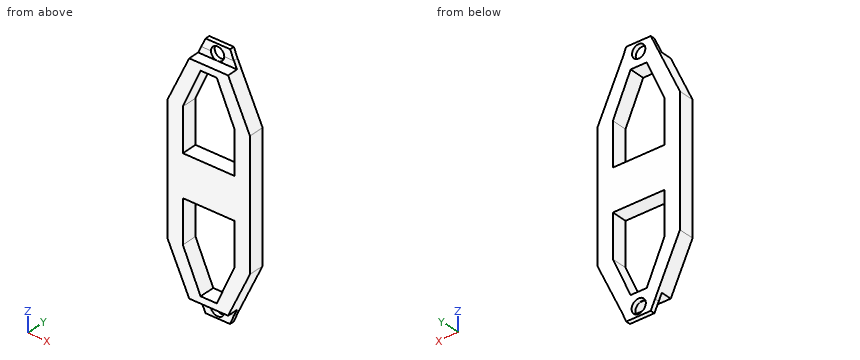
Autodesk Inventor part; units mm, degrees
ref_plane "YZ Plane" through (0, 0, 0) normal (1, 0, 0) x (0, 1, 0)
ref_plane "XZ Plane" through (0, 0, 0) normal (0, 1, 0) x (-1, 0, 0)
ref_plane "XY Plane" through (0, 0, 0) normal (0, 0, 1) x (1, 0, 0)
sketch "Sketch1" plane through (0, 0, 0) normal (0, 1, 0) x (-1, 0, 0)
  line L0 (0, -213.8682) -> (0, 213.8682)
  line L1 (20.1057, -144) -> (-20.1057, -144)
  line L2 (-50.827, -78.2337) -> (-50.827, 78.2337)
  line L3 (-20.1057, 144) -> (20.1057, 144)
  line L4 (50.773, 78.2337) -> (50.773, -78.2337)
  line L5 (158.1712, 0) -> (-85.66, 0)
  line L6 (50.773, 78.2337) -> (20.1057, 144)
  line L7 (50.773, 78.2337) -> (123.3381, 78.2337) construction
  line L8 (-50.827, 78.2337) -> (-20.1057, 144)
  line L9 (-20.1057, 144) -> (20.1057, 144)
  line L10 (31.723, 78.2337) -> (31.723, -78.2337)
  line L11 (-31.777, -78.2337) -> (-31.777, 78.2337)
  line L12 (-20.1057, -144) -> (20.1057, -144)
  line L13 (50.773, -78.2337) -> (20.1057, -144)
  line L14 (-50.827, -78.2337) -> (-20.1057, -144)
  line L15 (31.723, -25.4) -> (31.723, 25.4)
  line L16 (31.723, -25.4) -> (-31.777, -25.4)
  line L17 (31.723, 25.4) -> (-31.777, 25.4)
  line L18 (31.723, 78.2337) -> (9.9071, 127.5128)
  line L19 (-31.777, 78.2337) -> (-9.9611, 127.5128)
  line L20 (-9.9611, 127.5128) -> (9.9071, 127.5128)
  line L21 (50.773, 78.2337) -> (31.723, 78.2337)
  line L22 (-31.777, 78.2337) -> (-50.827, 78.2337)
  line L23 (31.723, -78.2337) -> (9.9071, -127.5128)
  line L24 (-31.777, -78.2337) -> (-9.9611, -127.5128)
  line L25 (-9.9611, -127.5128) -> (9.9071, -127.5128)
  line L26 (50.773, -78.2337) -> (31.723, -78.2337)
  line L27 (-31.777, -78.2337) -> (-50.827, -78.2337)
  point P0 (50.8, -140)
  point P1 (-50.8, 140)
  point P2 (-50.8, -140)
  dimension "d49" = 280
  dimension "d51" = 115
  dimension "d52" = 101.6
  dimension "d53" = 50.8
  dimension "d71" = 288
extrude "Extrusion1" add sketch "Sketch1" along normal blind 19.05 contours L1 L14 L27 L24 L25 L0 | L0 L25 L23 L26 L13 L1 | L16 L11 L5 L0 | L0 L5 L10 L16 | L26 L10 L5 L4 | L2 L5 L11 L27 | L5 L11 L17 L0 | L0 L17 L10 L5 | L5 L10 L21 L4 | L2 L22 L11 L5 | L21 L18 L20 L0 L3 L6 | L8 L3 L0 L20 L19 L22
sketch "Sketch9" plane through (50.827, 0, 78.2337) normal (1, 0, 0) x (0, 0, -1)
  line L0 (-65.7663, 19.05) -> (0, 19.05)
  line L1 (-65.7663, 19.05) -> (-65.7663, 0)
  line L2 (-65.7663, 0) -> (-65.7663, 19.05)
  line L3 (-65.7663, 9.525) -> (-52.4585, 9.525)
  line L4 (-65.7663, 13.4938) -> (-65.7663, 5.5563)
  line L5 (-65.7663, 19.05) -> (-77.0693, 19.05)
  line L6 (-65.7663, 19.05) -> (-54.4633, 19.05) construction
  line L7 (-65.7663, 13.4938) -> (-77.0693, 13.4937)
  line L8 (-77.0693, 13.4937) -> (-77.0693, 19.05)
  line L9 (-65.7663, 19.05) -> (-65.7663, 13.4938)
  line L10 (78.2337, -3.81) -> (78.2337, 22.86)
  line L11 (222.2337, 19.05) -> (233.5367, 19.05)
  line L12 (222.2337, 13.4938) -> (233.5367, 13.4937)
  line L13 (233.5367, 13.4937) -> (233.5367, 19.05)
  line L14 (222.2337, 19.05) -> (222.2337, 13.4938)
  point P0 (78.2337, 0)
  dimension "d55" = 7.9375
  dimension "d56" = 11.303
  dimension "d57" = 180
extrude "Extrusion9" add sketch "Sketch9" against normal up to surface (70.9326 mm away)
sketch "Sketch10" plane through (0, 19.05, 0) normal (0, 1, 0) x (1, 0, 0)
  line L0 (20.1057, -144) -> (50.827, -78.2337)
  line L1 (20.1057, -144) -> (15.3607, -155.303)
  line L2 (50.827, -155.303) -> (-20.1057, -155.303)
  line L3 (15.3607, -155.303) -> (50.53, -155.303)
  line L4 (50.827, -144) -> (20.1057, -144)
  line L5 (20.1057, -144) -> (50.827, -144)
  line L6 (50.827, -144) -> (50.827, -155.303)
  line L7 (50.827, -144) -> (50.827, -155.303)
  line L8 (50.827, -155.303) -> (50.827, -144)
  line L9 (50.827, -155.303) -> (15.3607, -155.303)
  line L10 (-71.093, 0) -> (71.147, 0)
  line L11 (20.1057, 144) -> (15.3607, 155.303)
  line L12 (15.3607, 155.303) -> (50.53, 155.303)
  line L13 (50.827, 144) -> (20.1057, 144)
  line L14 (20.1057, 144) -> (50.827, 144)
  line L15 (50.827, 144) -> (50.827, 155.303)
  line L16 (50.827, 144) -> (50.827, 155.303)
  line L17 (50.827, 155.303) -> (50.827, 144)
  line L18 (50.827, 155.303) -> (15.3607, 155.303)
  line L19 (-20.1057, -144) -> (-14.8343, -155.303)
  line L20 (-20.1057, -155.303) -> (-14.8343, -155.303)
  line L21 (-50.773, -78.2337) -> (-20.1057, -144)
  line L22 (-20.1057, -155.303) -> (-20.1057, -144)
  line L23 (-20.1057, 144) -> (-14.8343, 155.303)
  line L24 (-20.1057, 155.303) -> (-14.8343, 155.303)
  line L25 (-20.1057, 155.303) -> (-20.1057, 144)
  point P0 (0, 0)
extrude "Extrusion10" cut sketch "Sketch10" against normal up to surface (19.05 mm away)
ref_plane "Work Plane1" through (50.827, 5.5626, -144) normal (0, 1, 0) x (1, 0, 0)
sketch "Sketch13" plane through (0, 19.05, 0) normal (0, 1, 0) x (1, 0, 0)
  circle A0 centre (0, -144) radius 8.1915
  circle A1 centre (0, 144) radius 8.763
  line L0 (-71.093, 0) -> (71.147, 0)
  point P0 (0, 0)
  dimension "d68" = 16.383
  dimension "d69" = 17.526
  dimension "d70" = 288
extrude "Extrusion13" cut sketch "Sketch13" against normal up to surface (5.5562 mm away)
sketch "Sketch14" plane through (50.827, 0, 78.2337) normal (1, 0, 0) x (0, 0, -1)
  line L0 (-57.5748, 19.05) -> (-57.5748, 5.5626)
  line L1 (-57.5748, 19.05) -> (-57.5748, 5.5626)
  line L2 (-57.5748, 19.05) -> (-57.5748, 5.5626)
  line L3 (-65.7663, 13.4938) -> (-57.5748, 13.4938)
  line L4 (-57.5748, 5.5626) -> (-57.5748, 13.4938)
  line L5 (-65.7663, 0) -> (-65.7663, 13.4938)
  line L6 (78.2337, -3.81) -> (78.2337, 22.86)
  line L7 (222.2337, 13.4938) -> (214.0422, 13.4938)
  line L8 (214.0422, 5.5626) -> (214.0422, 13.4938)
  line L9 (222.2337, 5.5626) -> (222.2337, 13.4938)
  line L10 (-57.5748, 5.5626) -> (-57.5748, 0)
  line L11 (-65.7663, 0) -> (0, 0)
  line L12 (-57.5748, 0) -> (-65.7663, 0)
  line L13 (-65.7663, 0) -> (-65.7663, 13.4938)
  line L14 (-65.7663, 0) -> (-65.7663, 13.4938)
  line L15 (222.2337, 0) -> (222.2337, 13.4938)
  line L16 (222.2337, 5.5626) -> (222.2337, 0)
  line L17 (222.2337, 0) -> (213.1622, 0)
  line L18 (156.4673, 0) -> (222.2337, 0)
  line L19 (214.0422, 5.5626) -> (214.0422, 0)
  point P0 (78.2337, 0)
  point P1 (-65.7663, 5.5626)
extrude "Extrusion14" cut sketch "Sketch14" against normal through all
properties part number "Diff_BarV2"
Here's how the part is built. I have some questions about the finished solid (model axes, mm). Coordinates: 2 decimals unless noted, no trailing zeros. Order: outer loops, then holes, each group sorted by start corner. A loop starts at its lowest first (then second) coordinate and runs counter-clockwise, first axis right, second up. Notation, with made-up numbers: (78, -16) - (119, -16) arc R19 ccw to (119, -5) - close; hole circle Ø5 at (7, 55). An arc over 180 degrees is marked (long way). One line per question, with ' | ' between items. Start each with the question number.
1. If we section it at A-A (z = 35.5): Write out the boundary of the cut face in (x, y), and give its area (3 significant figures).
2. If we section it at B-B (x = -43): Write out the boundary of the cut face in (y, z).
3. Please list where these lines run through material, in increasing order: line 1 along Z through (x, y) = (0, 17.3); line 2 along X through (y, z) = (16.2, -144); line 3 along X through (y, z) = (15.55, 144). Write a range as [from, to].
4. I'm going to push flat-ended pins straight in: pin 1 Ø5 at (y, z) = (13.5, 99.5) entering from -X; pin 2 Ø21.5 at (x, z) = (0, 144) entering from +Y; pin 3 Ø4 at (x, y) = (10.5, 3) entering from +Z; pin 4 Ø5.5 at (x, y) = (2, 5.5) entering from -Z. Where does each tip first touch, or does it pass through?
Model answer:
1) outline: (-50.77, 0) - (-31.72, 0) - (-31.72, 19.05) - (-50.77, 19.05) - close; (31.78, 0) - (50.83, 0) - (50.83, 19.05) - (31.78, 19.05) - close | area: 726 mm²
2) outline: (0, -94.9) - (19.05, -94.9) - (19.05, 94.9) - (0, 94.9) - close
3) line 1: z = [-155.3, -152.76], [-135.24, -127.51], [-25.4, 25.4], [127.51, 135.81], [152.19, 155.3] | line 2: x = [-20.11, -8.76], [8.76, 20.11] | line 3: x = [-20.11, -8.19], [8.19, 20.11]
4) pin 1: stops at x = -42.02 | pin 2: stops at y = 19.05 | pin 3: stops at z = 135.81 | pin 4: stops at z = -135.81
